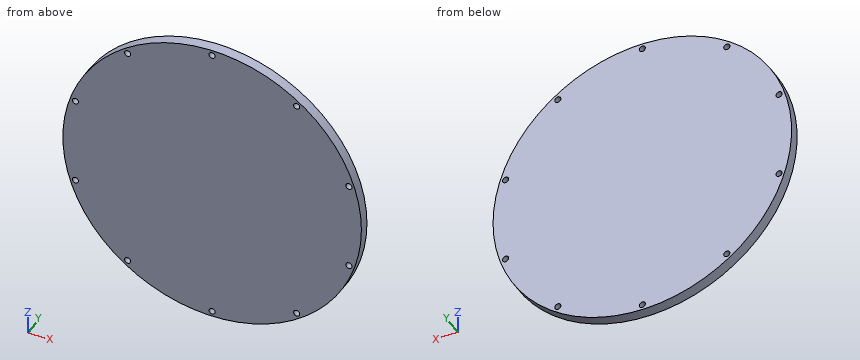
```python
from build123d import *

# Parameters (mm, degrees)
SKETCH1_R            = 82.55
BOSS_EXTRUDE1_DEPTH  = 3
M3_CLEARANCE_HOLE1_D = 3.4


with BuildPart() as part:
    # Sketch1 → Boss-Extrude1 (new body, symmetric)
    with BuildSketch(Plane(origin=(0, 0, 0), x_dir=(1, 0, 0), z_dir=(0, 1, 0))):
        Circle(SKETCH1_R)
    extrude(amount=BOSS_EXTRUDE1_DEPTH, both=True)

    # M3 Clearance Hole1 (through all)
    with Locations(Plane(origin=(0, 3, 0), x_dir=(1, 0, 0), z_dir=(0, 1, 0))):
        with Locations((0, 79.5), (46.728927557, 64.316851053), (75.608993045, 24.566851053), (75.608993045, -24.566851053), (46.728927557, -64.316851053), (0, -79.5), (-46.728927557, -64.316851053), (-75.608993045, -24.566851053), (-75.608993045, 24.566851053), (-46.728927557, 64.316851053)):
            Hole(M3_CLEARANCE_HOLE1_D / 2)


solid = part.part
```
Input: part model. Units: mm. Frame: model coordinates. Coordinates: 2 decimals unless noted, no trailing zeros. Loops run counter-clockwise (first coordinate to the right, second up) from the corner with the lowest first, then second, coordinate; pieces in that order, holes last.
Q1. Line query: line 1 along Z through (x, y) = (0, -0.15); line 2 along Z through (x, y) = (-0.5, -1.2); line 3 along X through (y, z) = (0.05, 24). Output: solid intervals per line, ascending.
Results are:
line 1: z = -82.55 to -81.2, -77.8 to 77.8, 81.2 to 82.55
line 2: z = -82.55 to -81.12, -77.88 to 77.88, 81.12 to 82.55
line 3: x = -78.98 to -77.21, -74.01 to 74.01, 77.21 to 78.98
Q2. Section C-C, the plane z = 32. Return the cut outline in (x, y).
Results are:
outline: (-76.1, -3) - (76.1, -3) - (76.1, 3) - (-76.1, 3) - close
Q3. Section A-A, the plane y = 0.7. Give the number of separate pieces and of enclosed holes in the cut face, and give its area (3 significant figures).
Results are:
separate pieces: 1
enclosed holes: 10
area: 21,300 mm2
Q4. Contact query for flat-ended pins moving along their axis: pin 1 (1.5 mm diameter, centred on y = -1.5, z = 39, fed in from -X); pin 2 (4.5 mm diameter, centred on x = 75.61, z = 24.57, fed in from +Y); pin 3 (3 mm diameter, centred on x = 17, y = 1, fed in from -Z). Output: stop coordinate, or through.
Results are:
pin 1: stops at x = -73.15
pin 2: stops at y = 3
pin 3: stops at z = -81.08
Q5. Section B-B, the plane x = -64. Return the cut outline in (y, z), and give its area (3 significant figures).
Results are:
outline: (-3, -52.14) - (3, -52.14) - (3, 52.14) - (-3, 52.14) - close
area: 626 mm2
